```python
from build123d import *

# Parameters (mm, degrees)
EXTRUDE_1_DEPTH     = 70
SKETCH_18_R         = 8
CUT_EXTRUDE_1_DEPTH = 9


with BuildPart() as part:
    # 草图1 → 凸台-拉伸1 (new body)
    with BuildSketch(Plane.XY):
        Polygon((-7, 23), (-7, -23), (10, -23), (10, -19.3), (9.175277675, -19.3), (8.8, -19.95), (5.2, -19.95), (5.2, -13.65), (8.8, -13.65), (9.175277675, -14.3), (10, -14.3), (10, 14.3), (9.175277675, 14.3), (8.8, 13.65), (5.2, 13.65), (5.2, 19.95), (8.8, 19.95), (9.175277675, 19.3), (10, 19.3), (10, 23), align=None)
    extrude(amount=-EXTRUDE_1_DEPTH)

    # 草图2 → 切除-旋转1 (revolve, cut)
    with BuildSketch(Plane(origin=(0, 0, 0), x_dir=(0, 0, -1), z_dir=(1, 0, 0))):
        Polygon((0, 10), (0, 13), (20, 13), (20, 15), (40, 15), (40, 10), align=None)
    revolve(axis=Axis((0, 10, -40), (0, 0, 1)), mode=Mode.SUBTRACT)

    # 草图3 → 切除-旋转2 (revolve, cut)
    with BuildSketch(Plane(origin=(0, 0, 0), x_dir=(0, 0, -1), z_dir=(1, 0, 0))):
        Polygon((0, -10), (0, -7), (20, -7), (20, -5), (40, -5), (40, -10), align=None)
    revolve(axis=Axis((0, -10, -40), (0, 0, 1)), mode=Mode.SUBTRACT)

    # 草图4 → 切除-旋转3 (revolve, cut)
    with BuildSketch(Plane.XY.offset(-20)):
        Polygon((-7, 0), (-7, 1.7), (6.7, 1.7), (6.7, 3.25), (10, 3.25), (10, 0), align=None)
    revolve(axis=Axis((10, 0, -20), (-1, 0, 0)), mode=Mode.SUBTRACT)

    # 草图5 → 切除-旋转4 (revolve, cut)
    with BuildSketch(Plane.XY.offset(-50)):
        Polygon((-7, 0), (-7, 1.7), (6.7, 1.7), (6.7, 3.25), (10, 3.25), (10, 0), align=None)
    revolve(axis=Axis((10, 0, -50), (-1, 0, 0)), mode=Mode.SUBTRACT)

    # 草图6 → 切除-旋转5 (revolve, cut)
    with BuildSketch(Plane.XY.offset(-20)):
        Polygon((-7, 0), (-7, 2), (-6.621, 1.621), (0, 1.621), (0.935884786, 0), align=None)
    revolve(axis=Axis((0.935884786, 0, -20), (-1, 0, 0)), mode=Mode.SUBTRACT)

    # 草图7 → 切除-旋转6 (revolve, cut)
    with BuildSketch(Plane.XY.offset(-50)):
        Polygon((-7, 0), (-7, 2), (-6.621, 1.621), (0, 1.621), (0.935884786, 0), align=None)
    revolve(axis=Axis((0.935884786, 0, -50), (-1, 0, 0)), mode=Mode.SUBTRACT)

    # 草图8 → 切除-旋转7 (revolve, cut)
    with BuildSketch(Plane(origin=(0, 0, 0), x_dir=(0, 0, -1), z_dir=(1, 0, 0))):
        Polygon((30, 17.306616994), (27.933, 18.5), (27.933, 22.567), (27.5, 23), (30, 23), align=None)
    revolve(axis=Axis((0, 23, -30), (0, -1, 0)), mode=Mode.SUBTRACT)

    # 草图9 → 切除-旋转8 (revolve, cut)
    with BuildSketch(Plane(origin=(0, 0, 0), x_dir=(0, 0, -1), z_dir=(1, 0, 0))):
        Polygon((62, 17.306616994), (59.933, 18.5), (59.933, 22.567), (59.5, 23), (62, 23), align=None)
    revolve(axis=Axis((0, 23, -62), (0, -1, 0)), mode=Mode.SUBTRACT)

    # 草图10 → 切除-旋转9 (revolve, cut)
    with BuildSketch(Plane(origin=(0, 0, 0), x_dir=(0, 0, -1), z_dir=(1, 0, 0))):
        Polygon((30, -23), (27.5, -23), (27.933, -22.567), (27.933, -18.5), (30, -17.306616994), align=None)
    revolve(axis=Axis((0, -17.306616994, -30), (0, -1, 0)), mode=Mode.SUBTRACT)

    # 草图11 → 切除-旋转10 (revolve, cut)
    with BuildSketch(Plane(origin=(0, 0, 0), x_dir=(0, 0, -1), z_dir=(1, 0, 0))):
        Polygon((62, -23), (59.5, -23), (59.933, -22.567), (59.933, -18.5), (62, -17.306616994), align=None)
    revolve(axis=Axis((0, -17.306616994, -62), (0, -1, 0)), mode=Mode.SUBTRACT)

    # 草图12 → 切除-旋转11 (revolve, cut)
    with BuildSketch(Plane(origin=(1.5, 0, 0), x_dir=(0, 0, -1), z_dir=(1, 0, 0))):
        Polygon((20, 17.790147844), (18.7705, 18.5), (18.7705, 22.7295), (18.5, 23), (20, 23), align=None)
    revolve(axis=Axis((1.5, 23, -20), (0, -1, 0)), mode=Mode.SUBTRACT)

    # 草图13 → 切除-旋转12 (revolve, cut)
    with BuildSketch(Plane(origin=(1.5, 0, 0), x_dir=(0, 0, -1), z_dir=(1, 0, 0))):
        Polygon((50, 17.790147844), (48.7705, 18.5), (48.7705, 22.7295), (48.5, 23), (50, 23), align=None)
    revolve(axis=Axis((1.5, 23, -50), (0, -1, 0)), mode=Mode.SUBTRACT)

    # 草图14 → 切除-旋转13 (revolve, cut)
    with BuildSketch(Plane(origin=(1.5, 0, 0), x_dir=(0, 0, -1), z_dir=(1, 0, 0))):
        Polygon((20, -23), (18.5, -23), (18.7705, -22.7295), (18.7705, -18.5), (20, -17.790147844), align=None)
    revolve(axis=Axis((1.5, -17.790147844, -20), (0, -1, 0)), mode=Mode.SUBTRACT)

    # 草图15 → 切除-旋转14 (revolve, cut)
    with BuildSketch(Plane(origin=(1.5, 0, 0), x_dir=(0, 0, -1), z_dir=(1, 0, 0))):
        Polygon((50, -23), (48.5, -23), (48.7705, -22.7295), (48.7705, -18.5), (50, -17.790147844), align=None)
    revolve(axis=Axis((1.5, -17.790147844, -50), (0, -1, 0)), mode=Mode.SUBTRACT)

    # 草图16 → 旋转1 (revolve)
    with BuildSketch(Plane(origin=(5, 0, 0), x_dir=(0, 0, -1), z_dir=(1, 0, 0))):
        Polygon((-3.2, 0), (-3.2, 3.5), (-2.262177826, 7), (-0.937822174, 7), (0, 3.5), (0, 0), align=None)
    revolve(axis=Axis((5, 0, 0), (0, 0, 1)))

    # 草图17 → 旋转2 (revolve)
    with BuildSketch(Plane(origin=(5, 0, 0), x_dir=(0, 0, -1), z_dir=(1, 0, 0))):
        Polygon((-9, 0), (-9, 3.5), (-8.062177826, 7), (-5.287822174, 7), (-4.35, 3.5), (-4.35, 2), (-3.2, 2), (-3.2, 0), align=None)
    revolve(axis=Axis((5, 0, 3.2), (0, 0, 1)))

    # 草图18 → 切除-拉伸1 (cut)
    with BuildSketch(Plane.XY):
        with Locations((5, 0)):
            Circle(SKETCH_18_R)
        Polygon((1.5, 2.020725942), (1.5, -2.020725942), (5, -4.041451884), (8.5, -2.020725942), (8.5, 2.020725942), (5, 4.041451884), align=None, mode=Mode.SUBTRACT)
    extrude(amount=CUT_EXTRUDE_1_DEPTH, mode=Mode.SUBTRACT)


solid = part.part
```
Can you work these out from the model? Positions are in its coordinate system, mm. A direction names the side the tool comes from. Coordinates: 2 decimals unless noted, no trailing zeros. Order: outer loops, then holes, each group sorted by start corner. A loop starts at its lowest first (then second) coordinate and runs counter-clockwise, first axis right, second up.
1. If we section it at B-B (y = 10): Please give me the cut outline in (x, z).
2. If we section it at A-A (z = -7.5): Please give me the cut outline in (x, y), then the cut area to 3 significant figures.
3. If we section it at C-C (z = -57): Please give me the cut outline in (x, y).
4. I need wall thicknesses on line 1 (Y direction, x = 6.25, z = -16.5); line 2 (Z direction, x = -3, y = 0); line 3 (X direction, y = -20.4, z = -50). Which ranges of each line are inside material? Lowest first, please.
5. Thinking about a two-plate mould opening in Y: for faces 6 (the face through (7, 13.65, -35)), 7 (the face through (1.5, 0, 7)), 8 (the face through (6.726, -3.045, 6.642)), which applies, +Y half, -Y half, draft (parallel to the pull), parting line (faces both ways), or undercut?
6. For faces 1 (the face through (6.8, 3, 6.6)), 2 (the face through (1.131, 20.644, -18.827)), 3 (the face through (-0.091, -20.505, -64.065)), 4 (the face through (8.19, -1.85, 4.4)), 5 (the face through (6.7, -1.4, -18.6)), which set-ups out of +Z, -Z, +X, -X, +Y, -Y let a thin tool reach every point of the face, with its end or its side?
7. I'm going to push flat-ended pins straight in: pin 1 (1.6 mm diameter, centred on y = 0, z = 2, fed in from -X); pin 2 (1.5 mm diameter, centred on x = 1.5, z = -20, fed in from +Y); pin 3 (3 mm diameter, centred on y = 16, z = -10.5, fed in from +X); pin 4 (2 mm diameter, centred on y = 0, z = -50, fed in from -X). Where does each tip first touch, or does it pass through?
8. If we section it at D-D (z = -39): Please give me the cut outline in (x, y), then the cut area to 3 significant figures.
Entries:
1. outline: (-7, -70) - (10, -70) - (10, 0) - (3, 0) - (3, -20) - (5, -20) - (5, -40) - (-5, -40) - (-5, -20) - (-3, -20) - (-3, 0) - (-7, 0) - close
2. outline: (-7, -23) - (10, -23) - (10, -19.3) - (9.18, -19.3) - (8.8, -19.95) - (5.2, -19.95) - (5.2, -13.65) - (8.8, -13.65) - (9.18, -14.3) - (10, -14.3) - (10, 14.3) - (9.18, 14.3) - (8.8, 13.65) - (5.2, 13.65) - (5.2, 19.95) - (8.8, 19.95) - (9.18, 19.3) - (10, 19.3) - (10, 23) - (-7, 23) - close; hole circle Ø6 at (0, -10); hole circle Ø6 at (0, 10)
2. area: 668 mm2
3. outline: (-7, -23) - (10, -23) - (10, -19.3) - (9.18, -19.3) - (8.8, -19.95) - (5.2, -19.95) - (5.2, -13.65) - (8.8, -13.65) - (9.18, -14.3) - (10, -14.3) - (10, 14.3) - (9.18, 14.3) - (8.8, 13.65) - (5.2, 13.65) - (5.2, 19.95) - (8.8, 19.95) - (9.18, 19.3) - (10, 19.3) - (10, 23) - (-7, 23) - close
4. line 1: y = -23 to -19.95, -13.65 to 13.65, 19.95 to 23
4. line 2: z = -70 to -51.7, -48.3 to -21.7, -18.3 to 0
4. line 3: x = -7 to 0.27, 2.73 to 10
5. face 6: undercut
5. face 7: draft
5. face 8: -Y half
6. face 1: +Z, +X, +Y
6. face 2: +Y
6. face 3: -Y
6. face 4: +X, -Y
6. face 5: +X
7. pin 1: stops at x = 1.5
7. pin 2: stops at y = 18.22
7. pin 3: stops at x = 5.2
7. pin 4: passes through
8. outline: (-7, -23) - (10, -23) - (10, -19.3) - (9.18, -19.3) - (8.8, -19.95) - (5.2, -19.95) - (5.2, -13.65) - (8.8, -13.65) - (9.18, -14.3) - (10, -14.3) - (10, 14.3) - (9.18, 14.3) - (8.8, 13.65) - (5.2, 13.65) - (5.2, 19.95) - (8.8, 19.95) - (9.18, 19.3) - (10, 19.3) - (10, 23) - (-7, 23) - close; hole circle Ø10 at (0, -10); hole circle Ø10 at (0, 10)
8. area: 567 mm2
